Input: part model. Units: mm. Frame: model coordinates. A direction names the side the tool comes from. Coordinates: 2 decimals unless noted, no trailing zeros. Write each loop counter-clockwise with the first axis right and the second up, starting at its lowest first coordinate (ties: lowest second). Pieces come first, ordered by that corner, then holes. Notation, with made-up numbers: (21, -22) - (29, -22) arc R10 cw to (29, -15) - close; hole circle Ø8 at (-9.75, -16). An arc over 180 degrees is marked (long way). Use CSV: the item, a comma, the result in double quotes.
```python
from build123d import *

# Parameters (mm, degrees)
SKETCH_1_W      = 18
SKETCH_1_H      = 14
EXTRUDE_1_DEPTH = 12
SKETCH_2_W      = 2.064874792
SKETCH_2_H      = 8.438190256
EXTRUDE_2_DEPTH = 5
FILLET_1_R      = 1


with BuildPart() as part:
    # Эскиз1 → Бобышка-Вытянуть1 (new body)
    with BuildSketch(Plane.XY):
        Rectangle(SKETCH_1_W, SKETCH_1_H)
    extrude(amount=EXTRUDE_1_DEPTH)

    # Эскиз2 → Бобышка-Вытянуть2 (add)
    with BuildSketch(Plane.XY.offset(12)):
        with Locations((-3.943253735, 0)):
            Rectangle(SKETCH_2_W, SKETCH_2_H)
    extrude(amount=EXTRUDE_2_DEPTH)

    # Скругление1
    fillet_1_edges = [part.edges().sort_by_distance(p)[0] for p in [
        (-9, 0, 12),
        (0, -7, 12),
        (9, 0, 12),
        (0, -7, 0),
        (-9, 0, 0),
        (0, 7, 0),
        (9, 0, 0),
        (0, 7, 12),
        (9, -7, 6),
        (-9, -7, 6),
        (-9, 7, 6),
        (9, 7, 6),
    ]]
    fillet(fillet_1_edges, radius=FILLET_1_R)


solid = part.part
```
(1) Cut plane C-C on z = 12.75. Return loops of the section in (x, y), and give its area (3 significant figures).
Check values:
outline,"(-4.98, -4.22) - (-2.91, -4.22) - (-2.91, 4.22) - (-4.98, 4.22) - close"
area,"17.4 mm^2"
(2) Pin query (flat end, axial travel): pin 1 Ø3 at (x, y) = (4, 2.5) entering from +Z; pin 2 Ø4 at (y, z) = (1.5, 15.5) entering from -X; pin 3 Ø1 at (x, z) = (-6.5, 12) entering from +Y. Return the tip coordinate at first contact, or that it passes through.
Check values:
pin 1,"z = 12"
pin 2,"x = -4.98"
pin 3,"y = 6.87"
(3) Cut plane A-A on y = -1.75. Return loops of the section in (x, z).
Check values:
outline,"(-9, 1) arc R1 ccw to (-8, 0) - (8, 0) arc R1 ccw to (9, 1) - (9, 11) arc R1 ccw to (8, 12) - (-2.91, 12) - (-2.91, 17) - (-4.98, 17) - (-4.98, 12) - (-8, 12) arc R1 ccw to (-9, 11) - close"
(4) Reachability of faces 1 (the cylindrical face through (8.699, 0.084, 0.285)), 2 (the flat face through (-4.976, 0, 14)), 3 (the flat face through (-4, -4.219, 14)), 4 (the flat face through (-2.911, 0, 14)), 5 (the flat face through (-4, 4.219, 14)) from +Z, -Z, +X, -X, +Y, -Y: full face, straight path, thin tool, end or side. Return the list, or none.
Check values:
face 1,"-Z, +X, +Y, -Y"
face 2,"+Z, -X, +Y, -Y"
face 3,"+Z, +X, -X, -Y"
face 4,"+Z, +X, +Y, -Y"
face 5,"+Z, +X, -X, +Y"
(5) Ray query, probe 1 along X at (y, z) = (-0.75, 14); probe 2 along Z at (x, y) = (-6.5, -2.75); probe 3 along Y at (x, z) = (-3, 12.5). Return the intervals inside material, ascending. Write a range as from..to.
Check values:
probe 1,"-4.98..-2.91"
probe 2,"0..12"
probe 3,"-4.22..4.22"
(6) Cut plane B-B on x = 7. Return loops of the section in (y, z).
Check values:
outline,"(-7, 1) arc R1 ccw to (-6, 0) - (6, 0) arc R1 ccw to (7, 1) - (7, 11) arc R1 ccw to (6, 12) - (-6, 12) arc R1 ccw to (-7, 11) - close"
(7) Draft query along X for faces 6 (the flat face through (-9, 0, 6)), 7 (the cylindrical face through (8.699, -6.715, 6.07)), 8 (the cylindrical face through (0.112, -6.715, 0.301)). Return one class per face: pulls with the +X half, pulls with the -X half, needs draft (parallel to the pull), parting line crosses it, or undercut.
Check values:
face 6,"pulls with the -X half"
face 7,"pulls with the +X half"
face 8,"needs draft"
